Design review of the part built by this model. Coordinates are the model's own, in mm. A direction names the side the tool comes from. Coordinates: 2 decimals unless noted, no trailing zeros. Loops run counter-clockwise (first coordinate to the right, second up) from the corner with the lowest first, then second, coordinate; pieces in that order, holes last. Notation, with made-up numbers: (7, -27.75) - (15, -27.75) arc R13 ccw to (15, -18.75) - close; hole circle Ø10 at (58.25, 41.25). An arc over 180 degrees is marked (long way). Answer in a Markdown table with one row per item. Add a question column.
(1) We need section A-A, the plane y = 107.5. Write out the cut boundary in (x, z).
(2) The part is to be moulded in two halves that separate along Y. For faces 3 (the face through (-46.609, 113, 227)), 4 (the face through (-43.434, 113, 227)), 5 (the face through (-33.03, 122.75, 440.98)), say which applies: released by +Y, released by -Y, zero draft, split by the parting line, or undercut.
(3) We need section B-B, the plane z = 56.5. Write out the cut boundary in (x, y).
(4) We need section C-C, the plane x = -32. Write out the cut boundary in (y, z) (3 decimals).
(5) For faces 1 (the face through (-34, 103.355, 227)), 2 (the face through (-34, 100.18, 227)), list the 3-axis set-ups (+Z, -Z, +X, -X, +Y, -Y) from which the entire face can be reached by the end or side of a thin tool; tool diameter is ignored.
(6) To check wall thickness, follow L1, parallel to Y at x = -33.5, z = 85; L2, parallel to X at y = 118.25, z = 301.5; L3, parallel to Z at x = -23.5, y = 111. State the ranges of each line that lie inside material, in increasing order. Write a range as [from, to].
Autodesk Inventor part; units mm, degrees
ref_plane "YZ Plane" through (0, 0, 0) normal (1, 0, 0) x (0, 1, 0)
ref_plane "XZ Plane" through (0, 0, 0) normal (0, 1, 0) x (-1, 0, 0)
ref_plane "XY Plane" through (0, 0, 0) normal (0, 0, 1) x (1, 0, 0)
sketch "Sketch1" plane through (0, 0, 0) normal (0, 0, 1) x (1, 0, 0)
  line L0 (-46.6093, 125.5803) -> (-21.2093, 125.5803)
  line L1 (-21.2093, 125.5803) -> (-21.2093, 100.1803)
  line L2 (-21.2093, 100.1803) -> (-46.6093, 100.1803)
  line L3 (-46.6093, 100.1803) -> (-46.6093, 125.5803)
  line L4 (-43.4343, 122.4053) -> (-24.3843, 122.4053)
  line L5 (-24.3843, 122.4053) -> (-24.3843, 103.3553)
  line L6 (-24.3843, 103.3553) -> (-43.4343, 103.3553)
  line L7 (-43.4343, 103.3553) -> (-43.4343, 122.4053)
  point P0 (0, 0)
  dimension "d0" = 25.4
  dimension "d1" = 25.4
  dimension "d2" = 3.175
extrude "Extrusion1" add sketch "Sketch1" along normal blind 460.375
sketch "Sketch2" plane through (-46.6093, 100.1803, 0) normal (-1, 0, 0) x (0, 0, 1)
  point P0 (0, -100.1803)
sketch "Sketch3" plane through (-46.6093, 100.1803, 0) normal (-1, 0, 0) x (0, 0, 1)
  point P0 (0, -100.1803)
chamfer "Chamfer1" distance 22.225 angle 45 2 edges at (-33.9093, 125.5803, 460.375) (-33.9093, 125.5803, 0)
properties part number "2018 Bottom Cross Bar"
Responses:
| question | item | result |
|---|---|---|
| 1 | outline | (-46.61, 4.14) - (-43.43, 4.14) - (-43.43, 456.23) - (-46.61, 456.23) - close; (-24.38, 4.14) - (-21.21, 4.14) - (-21.21, 456.23) - (-24.38, 456.23) - close |
| 2 | face 3 | zero draft |
| 2 | face 4 | undercut |
| 2 | face 5 | released by +Y |
| 3 | outline | (-46.61, 100.18) - (-21.21, 100.18) - (-21.21, 125.58) - (-46.61, 125.58) - close; hole (-43.43, 103.36) - (-24.38, 103.36) - (-24.38, 122.41) - (-43.43, 122.41) - close |
| 4 | outline | (100.18, 0) - (103.355, 0) - (103.355, 460.375) - (100.18, 460.375) - close; (122.405, 19.05) - (125.58, 22.225) - (125.58, 438.15) - (122.405, 441.325) - close |
| 5 | face 1 | +Z, -Z |
| 5 | face 2 | +Z, -Z, +X, -X, -Y |
| 6 | L1 | y = [100.18, 103.36], [122.41, 125.58] |
| 6 | L2 | x = [-46.61, -43.43], [-24.38, -21.21] |
| 6 | L3 | z = [7.64, 452.73] |
